Autodesk Inventor part; units mm, degrees
ref_plane "YZ Plane" through (0, 0, 0) normal (1, 0, 0) x (0, 1, 0)
ref_plane "XZ Plane" through (0, 0, 0) normal (0, 1, 0) x (-1, 0, 0)
ref_plane "XY Plane" through (0, 0, 0) normal (0, 0, 1) x (1, 0, 0)
sketch "Sketch1" plane through (0, 0, 0) normal (0, 1, 0) x (-1, 0, 0)
  line L0 (-14.666, -11.6564) -> (-8.516, -11.6564)
  line L1 (-8.516, -11.6564) -> (-8.516, -13.7564)
  line L2 (-8.516, -13.7564) -> (-14.666, -13.7564)
  line L3 (-14.666, -13.7564) -> (-14.666, -11.6564)
  line L4 (-14.666, -11.6564) -> (-8.516, -13.7564) construction
  line L5 (-8.516, -11.6564) -> (-14.666, -13.7564) construction
  line L6 (-16.166, -15.2564) -> (-7.016, -15.2564)
  line L7 (-7.016, -15.2564) -> (-7.016, -10.1564)
  line L8 (-16.166, -10.1564) -> (-16.166, -15.2564)
  line L9 (-16.166, -8.1564) -> (-7.016, -8.1564)
  line L10 (-7.016, -10.1564) -> (-7.016, -8.1564)
  line L11 (-16.166, -10.1564) -> (-16.166, -8.1564)
  point P0 (0, 0)
  point P1 (-11.591, -12.7064)
  dimension "d0" = 6.15
  dimension "d1" = 2.1
  dimension "d2" = 1.5
extrude "Extrusion1" add sketch "Sketch1" along normal blind 8
sketch "Sketch4" plane through (7.016, 0, -8.1564) normal (0, 0, 1) x (1, 0, 0)
  circle A0 centre (4.5664, 4) radius 1.15
  point P0 (-7.016, 0)
  dimension "d13" = 2.3
extrude "Extrusion4" cut sketch "Sketch4" against normal blind 4
sketch "Sketch5" plane through (16.166, 0, -15.2564) normal (0, 0, -1) x (-1, 0, 0)
  line L0 (2.3524, 6.0027) -> (6.3524, 6.0027)
  line L1 (6.3524, 6.0027) -> (6.3524, 8.0027)
  line L2 (6.3524, 8.0027) -> (2.3524, 8.0027)
  line L3 (2.3524, 8.0027) -> (2.3524, 6.0027)
  line L4 (2.3524, 6.0027) -> (6.3524, 8.0027) construction
  line L5 (6.3524, 6.0027) -> (2.3524, 8.0027) construction
  point P0 (16.166, 0)
  point P1 (4.3524, 7.0027)
  dimension "d16" = 4
  dimension "d17" = 2
extrude "Extrusion5" add sketch "Sketch5" along normal blind 25
fillet "Fillet1" radius 1 3 edges at (11.8136, 6.0027, -15.2564) (9.8136, 7.0014, -15.2564) (13.8136, 7.0014, -15.2564)
thread "Thread1"
properties part number "slider"
Input: part model. Units: mm. Frame: model coordinates. A direction names the side the tool comes from. Coordinates: 2 decimals unless noted, no trailing zeros. Loops run counter-clockwise (first coordinate to the right, second up) from the corner with the lowest first, then second, coordinate; pieces in that order, holes last.
(1) Section D-D on x = 12. Count the separate pieces of the cut face and the enclosed holes in it, then the cut area to 3 significant figures.
(2) Section C-C on y = 4. Return the cut outline in (x, z).
(3) Set-up query: faces 4 (the face through (13.814, 7, -28)), 5 (the face through (10.735, 4.777, -9.882)), 6 (the face through (12, 6.003, -28)), 7 (the face through (12, 4, -13.756)). Return all of +Z, -Z, +X, -X, +Y, -Y with unobstructed straight access to the full face (end or side cutting, diameter ignored); none if empty.
(4) Section B-B on z = -12. Return the cut outline in (x, y), then the cut area to 3 significant figures.
(5) Pull-direction query (X, two-part tool) for faces 1 (the face through (9.814, 7, -28)), 2 (the face through (13, 4, -11.656)), 3 (the face through (12, 7, -40.256)); classes: released by +X, released by -X, zero draft, split by the parting line, or undercut.
(6) Material intervals for probe 1 along Z at (x, y) = (11, 6.5); probe 2 along Z at (x, y) = (13.75, 4); probe 3 along Y at (x, z) = (10.25, -37), sorted ascending.
(7) First-contact query: pin 1 Ø3 at (x, z) = (12.5, -23.5) entering from -Y; pin 2 Ø2 at (x, y) = (11.58, 4) entering from +Z; pin 3 Ø0.6 at (y, z) = (7.5, -28.5) entering from +X. Flat tips, straight axial feed; report the tip coordinate or a pass-through.
Data:
1. separate pieces: 3
1. enclosed holes: 0
1. area: 82.7 mm2
2. outline: (7.02, -15.26) - (16.17, -15.26) - (16.17, -8.16) - (12.73, -8.16) - (12.73, -11.66) - (14.67, -11.66) - (14.67, -13.76) - (8.52, -13.76) - (8.52, -11.66) - (10.43, -11.66) - (10.43, -8.16) - (7.02, -8.16) - close
3. face 4: -Z, +X, +Y, -Y
3. face 5: +Z
3. face 6: -Z, +X, -X, -Y
3. face 7: +Y, -Y
4. outline: (7.02, 0) - (8.52, 0) - (8.52, 8) - (7.02, 8) - close; (14.67, 0) - (16.17, 0) - (16.17, 8) - (14.67, 8) - close
4. area: 24.0 mm2
5. face 1: released by -X
5. face 2: undercut
5. face 3: zero draft
6. probe 1: z = -40.26 to -13.76, -11.66 to -8.16
6. probe 2: z = -15.26 to -13.76, -11.66 to -8.16
6. probe 3: y = 6 to 8
7. pin 1: stops at y = 6
7. pin 2: stops at z = -13.76
7. pin 3: stops at x = 13.81
